Geometry check sheet. Reference: the model listing, model coordinates, mm. A direction names the side the tool comes from. Coordinates: 2 decimals unless noted, no trailing zeros. Write each loop counter-clockwise with the first axis right and the second up, starting at its lowest first coordinate (ties: lowest second). Pieces come first, ordered by that corner, then holes. Notation, with made-up numbers: (28.25, 45) -> (38.25, 45) arc R20 ccw to (38.25, 70) -> close; hole circle Ø6 at (27, 56.5). An arc over 180 degrees is marked (long way). Answer in a Markdown table with one row per item. Add a question column.
1. Scan lines: L1, parallel to X at y = -4.25, z = -12.7; L2, parallel to X at y = -5, z = -11.5; L3, parallel to Z at x = 8.5, y = -1.25. Record each from-to range of solid material in increasing order. Write a range as from..to.
2. Cross-section at C-C on z = 31. Record the cut outline in (x, y).
3. Cross-section at A-A on y = -2. Record the cut outline in (x, z).
4. Mould release check, pull along X, two halves, no side actions. Record for faces 4 (the flat face through (16, -3, 12.7)), 5 (the cylindrical face through (36.01, -3.13, -21.43)): pulls with the +X half, pulls with the -X half, needs draft (parallel to the pull), parting line crosses it, or undercut.
5. Set-up check for faces 1 (the flat face through (-16, -3, 12.7)), 2 (the flat face through (-2.902, -3.131, -20.374)), 3 (the flat face through (-12, -6.35, -1)): record each of +Z, -Z, +X, -X, +Y, -Y from which the full face is reachable in a straight line by a thin tool's end or side.
6. Cross-section at D-D on z = -20. Record the cut outline in (x, y).
7. Cross-section at B-B on x = 7. Record the cut outline in (y, z), and give its area (3 significant figures).
8. Depth check by flat-ended pin: P1, Ø17.5, axis at x = -22, z = -12.7, coming from the +Y side; P2, Ø1.9, axis at x = 14.5, y = -3.5, coming from the +Z side; P3, Ø1.5, axis at x = -11, y = -1.5, coming from the -Z side; P4, Ø1.5, axis at y = -3, z = 27.5, coming from the -X side. Enter the tip coordinate at first touch or a pass-through.
```python
from build123d import *

# Parameters (mm, degrees)
F1_DEPTH = 6.35


with BuildPart() as f1:
    # F0 (on Front) → F1 (new body)
    with BuildSketch(Plane.XZ):
        with BuildLine():
            ThreePointArc((-5.723816, -15.486059), (-5.488792, -12.459869), (-5.811737, -9.441795))
            ThreePointArc((-5.811737, -9.441795), (-7.949382, -7.728591), (-9.60171, -5.54355))
            ThreePointArc((-9.60171, -5.54355), (-10.667847, -3.020071), (-11.082703, -0.312214))
            ThreePointArc((-11.082703, -0.312214), (-13.533332, 1.47553), (-16.269675, 2.784745))
            ThreePointArc((-16.269675, 2.784745), (-36.296072, -20.953359), (-5.723816, -15.486059))
        make_face()
        with BuildLine():
            ThreePointArc((-10.909945, -12.7), (-32.706361, -15.569553), (-12.395335, -7.15645))
            ThreePointArc((-12.395335, -7.15645), (-11.287729, -9.830447), (-10.909945, -12.7))
        make_face(mode=Mode.SUBTRACT)
        with BuildLine():
            ThreePointArc((16.267047, 2.783773), (13.532129, 1.474812), (11.082703, -0.312214))
            ThreePointArc((11.082703, -0.312214), (10.667847, -3.020071), (9.60171, -5.54355))
            ThreePointArc((9.60171, -5.54355), (7.949382, -7.728591), (5.811737, -9.441795))
            ThreePointArc((5.811737, -9.441795), (5.488694, -12.46668), (5.726121, -15.499486))
            ThreePointArc((5.726121, -15.499486), (36.300176, -20.946245), (16.267047, 2.783773))
        make_face()
        with BuildLine():
            ThreePointArc((33.084145, -12.7), (19.127493, -23.409316), (12.395335, -7.15645))
            ThreePointArc((12.395335, -7.15645), (24.866598, -1.990684), (33.084145, -12.7))
        make_face(mode=Mode.SUBTRACT)
        with BuildLine():
            ThreePointArc((0, 11.0871), (2.718465, 10.748662), (5.270966, 9.75401))
            ThreePointArc((5.270966, 9.75401), (8.046167, 10.983368), (10.549412, 12.7))
            ThreePointArc((10.549412, 12.7), (0, 41.91), (-10.549412, 12.7))
            ThreePointArc((-10.549412, 12.7), (-8.046167, 10.983368), (-5.270966, 9.75401))
            ThreePointArc((-5.270966, 9.75401), (-2.718465, 10.748662), (0, 11.0871))
        make_face()
        with BuildLine():
            ThreePointArc((11.0871, 25.4), (7.839764, 17.560236), (0, 14.3129))
            ThreePointArc((0, 14.3129), (-7.839764, 33.239764), (11.0871, 25.4))
        make_face(mode=Mode.SUBTRACT)
        with BuildLine():
            ThreePointArc((5.270966, 9.75401), (7.728591, 7.949382), (9.60171, 5.54355))
            Line((9.60171, 5.54355), (21.997045, 12.7))
            Line((21.997045, 12.7), (10.549412, 12.7))
            ThreePointArc((10.549412, 12.7), (8.046167, 10.983368), (5.270966, 9.75401))
        make_face()
        with BuildLine():
            ThreePointArc((9.60171, 5.54355), (10.709316, 2.869553), (11.0871, 0))
            ThreePointArc((11.0871, 0), (11.086001, -0.156123), (11.082703, -0.312214))
            ThreePointArc((11.082703, -0.312214), (13.532129, 1.474812), (16.267047, 2.783773))
            Line((16.267047, 2.783773), (21.997045, 12.7))
            Line((21.997045, 12.7), (9.60171, 5.54355))
        make_face()
        with BuildLine():
            ThreePointArc((5.726121, -15.499486), (5.488694, -12.46668), (5.811737, -9.441795))
            ThreePointArc((5.811737, -9.441795), (3.020071, -10.667847), (0, -11.0871))
            Line((0, -11.0871), (0, -25.4))
            Line((0, -25.4), (5.726121, -15.499486))
        make_face()
        with BuildLine():
            Line((0, -25.4), (0, -11.0871))
            ThreePointArc((0, -11.0871), (-3.020071, -10.667847), (-5.811737, -9.441795))
            ThreePointArc((-5.811737, -9.441795), (-5.488792, -12.459869), (-5.723816, -15.486059))
            Line((-5.723816, -15.486059), (0, -25.4))
        make_face()
        with BuildLine():
            ThreePointArc((-11.082703, -0.312214), (-10.748662, 2.718465), (-9.60171, 5.54355))
            Line((-9.60171, 5.54355), (-21.997045, 12.7))
            Line((-21.997045, 12.7), (-16.269675, 2.784745))
            ThreePointArc((-16.269675, 2.784745), (-13.533332, 1.47553), (-11.082703, -0.312214))
        make_face()
        with BuildLine():
            ThreePointArc((-9.60171, 5.54355), (-7.728591, 7.949382), (-5.270966, 9.75401))
            ThreePointArc((-5.270966, 9.75401), (-8.046167, 10.983368), (-10.549412, 12.7))
            Line((-10.549412, 12.7), (-21.997045, 12.7))
            Line((-21.997045, 12.7), (-9.60171, 5.54355))
        make_face()
    extrude(amount=F1_DEPTH)


solid = f1.part
```
Results found:
| question | item | result |
|---|---|---|
| 1 | L1 | x = -38.51..-33.08, -10.91..10.91, 33.08..38.51 |
| 1 | L2 | x = -38.46..-33.02, -10.98..10.98, 33.02..38.46 |
| 1 | L3 | z = -22.21..-7.12, 7.12..18.28, 32.52..39.55 |
| 2 | outline | (-15.53, -6.35) -> (-9.57, -6.35) -> (-9.57, 0) -> (-15.53, 0) -> close; (9.57, -6.35) -> (15.53, -6.35) -> (15.53, 0) -> (9.57, 0) -> close |
| 3 | outline | (-22, 12.7) -> (-16.27, 2.78) arc R16.51 ccw (long way) to (-5.72, -15.49) -> (0, -25.4) -> (5.73, -15.5) arc R16.51 ccw (long way) to (16.27, 2.78) -> (22, 12.7) -> (10.55, 12.7) arc R16.51 ccw (long way) to (-10.55, 12.7) -> close; hole circle Ø22.17 at (-22, -12.7); hole (-11.08, -0.31) arc R11.09 ccw to (-9.6, -5.54) arc R11.09 ccw to (-5.81, -9.44) arc R11.09 ccw to (0, -11.09) arc R11.09 ccw to (5.81, -9.44) arc R11.09 ccw to (9.6, -5.54) arc R11.09 ccw to (11.08, -0.31) arc R11.08 ccw to (11.09, 0) arc R11.09 ccw to (9.6, 5.54) arc R11.09 ccw to (5.27, 9.75) arc R11.09 ccw to (0, 11.09) arc R11.09 ccw to (-5.27, 9.75) arc R11.09 ccw to (-9.6, 5.54) arc R11.09 ccw to start; hole (0, 14.31) arc R11.09 ccw to (11.09, 25.4) arc R11.09 ccw (long way) to start; hole circle Ø22.17 at (22, -12.7) |
| 4 | face 4 | needs draft |
| 4 | face 5 | undercut |
| 5 | face 1 | -X, +Y, -Y |
| 5 | face 2 | -Z, +Y, -Y |
| 5 | face 3 | +Z, -Z, +X, -X, -Y |
| 6 | outline | (-36.81, -6.35) -> (-30.34, -6.35) -> (-30.34, 0) -> (-36.81, 0) -> close; (-13.65, -6.35) -> (-7.19, -6.35) -> (-7.19, 0) -> (-13.65, 0) -> close; (-3.12, -6.35) -> (3.12, -6.35) -> (3.12, 0) -> (-3.12, 0) -> close; (7.19, -6.35) -> (13.65, -6.35) -> (13.65, 0) -> (7.19, 0) -> close; (30.34, -6.35) -> (36.81, -6.35) -> (36.81, 0) -> (30.34, 0) -> close |
| 7 | outline | (-6.35, -19.6) -> (0, -19.6) -> (0, -8.6) -> (-6.35, -8.6) -> close; (-6.35, 8.6) -> (0, 8.6) -> (0, 16.8) -> (-6.35, 16.8) -> close; (-6.35, 34) -> (0, 34) -> (0, 40.35) -> (-6.35, 40.35) -> close |
| 7 | area | 162 mm^2 |
| 8 | P1 | passes through |
| 8 | P2 | stops at z = 34.83 |
| 8 | P3 | stops at z = -25.65 |
| 8 | P4 | stops at x = -16.45 |
